Read the model definition and answer for the solid it produces. Units are mm, in the model's axes. Face numbers are marked on the shaded views. A direction names the side the tool comes from. Coordinates: 2 decimals unless noted, no trailing zeros. Write each loop counter-clockwise with the first axis right and the second up, starting at its lowest first coordinate (ties: lowest second). Pieces come first, ordered by that corner, then holes.
1) The part is cut by section A-A (x = 8.5). Determine the outline of the cut face in (y, z), then the cut area to 3 significant figures.
2) The part is cut by section D-D (z = 12.5). Determine the outline of the cut face in (x, y), then the cut area to 3 significant figures.
3) The part is cut by section B-B (z = 0). Give the number of separate pieces and of enclosed holes in the cut face, then the cut area to 3 significant figures.
4) Which of the six approach directions +Z, -Z, +X, -X, +Y, -Y give full straight-line access (tool end or side, diameter ignored) to the marked faces 1, 2 and 3?
5) The part is cut by section C-C (y = 7.5). Determine the outline of the cut face in (x, z).
6) Find the intervals of material crossed by line 1 (X direction, y = 1.6, z = 0); line 2 (X direction, y = 4.5, z = -3); line 3 (Y direction, x = 6.75, z = 11.75), in increasing order.
7) Each of these flat-tipped pins is pushed along its axis until it touches: pin 1 Ø1 at (x, y) = (4.5, 7.5) entering from +Z; pin 2 Ø8 at (y, z) = (4, 6) entering from -X; pin 3 Ø3 at (y, z) = (2, 0.5) entering from +X; pin 4 Ø5 at (x, z) = (10, 0) entering from +Y. Where does it stop, or does it pass through?
8) Determine the mould class of the marked faces 4, 5, 6 and 7 for opening direction Z: +Z half, -Z half, draft (parallel to the pull), parting line (faces both ways), or undercut.
from build123d import *

# Parameters (mm, degrees)
SKETCH_1_R          = 15
EXTRUDE_1_DEPTH     = 5
SKETCH_2_R          = 1.9
CUT_EXTRUDE_1_DEPTH = 5
CUT_EXTRUDE_2_DEPTH = 2
SKETCH_4_R          = 5
EXTRUDE_2_DEPTH     = 10
FILLET_1_R          = 2
SKETCH_5_R          = 1.5
CUT_EXTRUDE_3_DEPTH = 15
CUT_EXTRUDE_4_DEPTH = 2.7


with BuildPart() as part:
    # Эскиз1 → Бобышка-Вытянуть1 (new body)
    with BuildSketch(Plane(origin=(0, 0, 0), x_dir=(1, 0, 0), z_dir=(0, 1, 0))):
        with Locations(Location((0, 0, 0), (0, 0, 270))):
            Circle(SKETCH_1_R)
    extrude(amount=EXTRUDE_1_DEPTH)

    # Эскиз2 → Вырез-Вытянуть1 (cut)
    with BuildSketch(Plane(origin=(0, 5, 0), x_dir=(1, 0, 0), z_dir=(0, 1, 0))):
        with Locations(Location((-10, 0, 0), (0, 0, 270))):
            Circle(SKETCH_2_R)
        with Locations(Location((10, 0, 0), (0, 0, 270))):
            Circle(SKETCH_2_R)
    extrude(amount=-CUT_EXTRUDE_1_DEPTH, mode=Mode.SUBTRACT)

    # Эскиз3 → Вырез-Вытянуть2 (cut)
    with BuildSketch(Plane(origin=(0, 5, 0), x_dir=(1, 0, 0), z_dir=(0, 1, 0))):
        Polygon((-10, -3.5), (-6.968911087, -1.75), (-6.968911087, 1.75), (-10, 3.5), (-13.031088913, 1.75), (-13.031088913, -1.75), align=None)
        Polygon((10, -3.5), (13.031088913, -1.75), (13.031088913, 1.75), (10, 3.5), (6.968911087, 1.75), (6.968911087, -1.75), align=None)
    extrude(amount=-CUT_EXTRUDE_2_DEPTH, mode=Mode.SUBTRACT)

    # Эскиз4 → Бобышка-Вытянуть2 (add)
    with BuildSketch(Plane(origin=(0, 5, 0), x_dir=(1, 0, 0), z_dir=(0, 1, 0))):
        with Locations(Location((0, 0, 0), (0, 0, 270))):
            Circle(SKETCH_4_R)
    extrude(amount=EXTRUDE_2_DEPTH)

    # Скругление1
    fillet_1_edges = [part.edges().sort_by_distance(p)[0] for p in [
        (0, 5, -5),
        (0, 15, -5),
    ]]
    fillet(fillet_1_edges, radius=FILLET_1_R)

    # Эскиз5 → Вырез-Вытянуть3 (cut)
    with BuildSketch(Plane.XZ):
        with Locations(Location((0, 0, 0), (0, 0, 270))):
            Circle(SKETCH_5_R)
    extrude(amount=-CUT_EXTRUDE_3_DEPTH, mode=Mode.SUBTRACT)

    # Эскиз6 → Вырез-Вытянуть4 (cut)
    with BuildSketch(Plane.XZ):
        Polygon((0, 3.5), (-3.031088913, 1.75), (-3.031088913, -1.75), (0, -3.5), (3.031088913, -1.75), (3.031088913, 1.75), align=None)
    extrude(amount=-CUT_EXTRUDE_4_DEPTH, mode=Mode.SUBTRACT)


solid = part.part
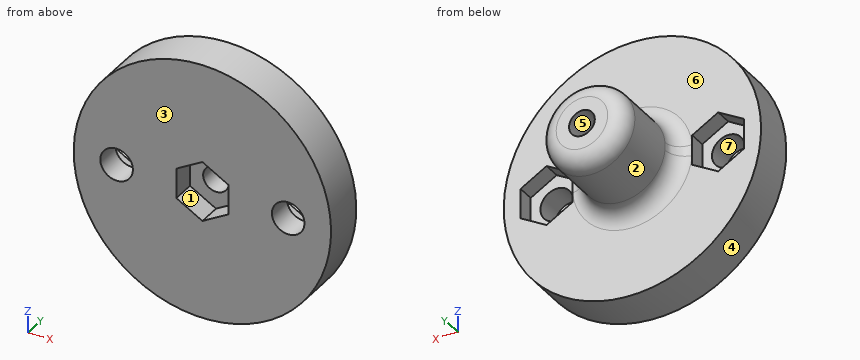
Reported:
1. outline: (0, -12.36) - (5, -12.36) - (5, -2.63) - (3, -2.63) - (3, -1.17) - (0, -1.17) - close; (0, 1.17) - (3, 1.17) - (3, 2.63) - (5, 2.63) - (5, 12.36) - (0, 12.36) - close
1. area: 106 mm2
2. outline: (-8.29, 0) - (8.29, 0) - (8.29, 5) - (-8.29, 5) - close
2. area: 82.9 mm2
3. separate pieces: 4
3. enclosed holes: 0
3. area: 150 mm2
4. face 1: -Y
4. face 2: +Y
4. face 3: +Z, -Z, +X, -X, -Y
5. outline: circle Ø10 at (0, 0); hole circle Ø3 at (0, 0)
6. line 1: x = -15 to -11.9, -8.1 to -3.03, 3.03 to 8.1, 11.9 to 15
6. line 2: x = -14.7 to -10.87, -9.13 to 9.13, 10.87 to 14.7
6. line 3: y = 0 to 5
7. pin 1: stops at z = 3
7. pin 2: stops at x = -14.87
7. pin 3: stops at x = 15
7. pin 4: stops at y = 3
8. face 4: parting line
8. face 5: undercut
8. face 6: draft
8. face 7: undercut
